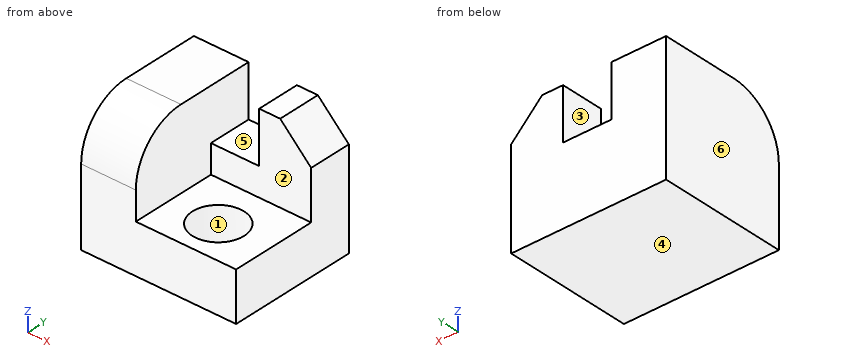
from build123d import *

# Parameters (mm, degrees)
F0_W     = 152.4
F0_H     = 127
F1_DEPTH = 127
F3_DEPTH = 78.74
F2_W     = 47.5228335708
F2_H     = 42.4285548031
F4_DEPTH = 50.8
F5_SIZE  = 30.48
F6_R     = 25.4
F7_DEPTH = 38.1
F8_R     = 50.8


with BuildPart() as f1:
    # F0 (on Top) → F1 (new body)
    with BuildSketch(Plane.XY):
        Rectangle(F0_W, F0_H)
    extrude(amount=F1_DEPTH)

    # F2 (on face) → F3 (cut)
    with BuildSketch(Plane.XY.offset(127)):
        Polygon((-22.4164314568, -24.2097526789), (-22.4164314568, -63.5), (76.2, -63.5), (76.2, 21.0714451969), (40.7979153097, 21.0714451969), (25.106402114, 21.0714451969), (-22.4164314568, 21.0714451969), align=None)
    extrude(amount=-F3_DEPTH, mode=Mode.SUBTRACT)

    # F2 (on face) → F4 (cut)
    with BuildSketch(Plane.XY.offset(127)):
        with Locations((1.3449853286, 42.2857225984)):
            Rectangle(F2_W, F2_H)
    extrude(amount=-F4_DEPTH, mode=Mode.SUBTRACT)

    # F5
    f5_edges = [f1.edges().sort_by_distance(p)[0] for p in [
        (76.2, 42.285723, 127),
    ]]
    chamfer(f5_edges, length=F5_SIZE)

    # F6 (on face) → F7 (cut)
    with BuildSketch(Plane.XY.offset(48.26)):
        with Locations((25.4, -25.4)):
            Circle(F6_R)
    extrude(amount=-F7_DEPTH, mode=Mode.SUBTRACT)

    # F8
    f8_edges = [f1.edges().sort_by_distance(p)[0] for p in [
        (-49.308216, -63.5, 127),
    ]]
    fillet(f8_edges, radius=F8_R)


solid = f1.part
Check sheet for the modelled part. Datum: model origin and axes. Units: mm. Face numbers are marked on the shaded views. A direction names the side the tool comes from. Round coordinates to 2 decimals unless told otherwise and drop trailing zeros. Loops run counter-clockwise (first coordinate to the right, second up) from the corner with the lowest first, then second, coordinate; pieces in that order, holes last.
1. Sectioned sample at A-A on y = 53.5. Record the boundary of the cut face in (x, z), and give its area (3 significant figures).
2. Mould release check, pull along X, two halves, no side actions. Record for the marked faces 4, 5 and 6: released by +X, released by -X, zero draft, split by the parting line, or undercut.
3. Set-up check for the marked faces 1, 2 and 3: record each of +Z, -Z, +X, -X, +Y, -Y from which the full face is reachable in a straight line by a thin tool's end or side.
4. Sectioned sample at B-B on x = 56. Record the boundary of the cut face in (y, z), and give its area (3 significant figures).
5. Sectioned sample at D-D on x = -34. Record the boundary of the cut face in (y, z).
6. Gauge pin test, flat ends, axial feed: pin 1 Ø1.5 at (x, y) = (-42.5, -36) entering from -Z; pin 2 Ø15 at (x, y) = (30, -30) entering from +Z; pin 3 Ø3 at (y, z) = (-26, 80.5) entering from +X. Record the tip position at first contact, or that the pin passes through.
7. Scan lines: probe 1 along Y at (x, z) = (25.4, 40); probe 2 along X at (y, z) = (-25, 25); probe 3 along X at (y, z) = (-3.5, 77.5). Record each from-to range of solid material in increasing order.
8. Sectioned sample at C-C on z = 14. Record the boundary of the cut face in (x, y), and give its area (3 significant figures).
Recorded:
1. outline: (-76.2, 0) - (76.2, 0) - (76.2, 96.52) - (45.72, 127) - (25.11, 127) - (25.11, 76.2) - (-22.42, 76.2) - (-22.42, 127) - (-76.2, 127) - close
1. area: 16,500 mm2
2. face 4: zero draft
2. face 5: undercut
2. face 6: released by -X
3. face 1: +Z
3. face 2: +Z, +X, -Y
3. face 3: +Z, +Y, -Y
4. outline: (-63.5, 0) - (63.5, 0) - (63.5, 116.72) - (21.07, 116.72) - (21.07, 48.26) - (-63.5, 48.26) - close
4. area: 9,030 mm2
5. outline: (-63.5, 0) - (63.5, 0) - (63.5, 127) - (-12.7, 127) arc R50.8 ccw to (-63.5, 76.2) - close
6. pin 1: stops at z = 0
6. pin 2: stops at z = 10.16
6. pin 3: stops at x = -22.42
7. probe 1: y = -63.5 to -50.8, 0 to 63.5
7. probe 2: x = -76.2 to 0, 50.8 to 76.2
7. probe 3: x = -76.2 to -22.42
8. outline: (-76.2, -63.5) - (76.2, -63.5) - (76.2, 63.5) - (-76.2, 63.5) - close; hole circle Ø50.8 at (25.4, -25.4)
8. area: 17,300 mm2
